Design review of the part built by this model. Coordinates are the model's own, in mm. Coordinates: 2 decimals unless noted, no trailing zeros. Write each loop counter-clockwise with the first axis right and the second up, starting at its lowest first coordinate (ties: lowest second). Pieces come first, ordered by that corner, then holes. Notation, with made-up numbers: (34.5, 3) - (70.5, 3) arc R28 ccw to (70.5, 21) - close; hole circle Ø8 at (10, -28.5). An arc over 180 degrees is marked (long way). Use a Markdown table: item, result.
from build123d import *

# Parameters (mm, degrees)
F1_DEPTH = 18
F3_D     = 8
F3_DEPTH = 11
F3_TIP   = 2.4034424761


# Not quite as in the source:
# - a feature names something its author has since deleted; it is built from what else it names


with BuildPart() as f1:
    # F0 (on Top) → F1 (new body)
    with BuildSketch(Plane.XY):
        with BuildLine():
            ThreePointArc((287.0371856283, 264.0258587081), (16.2714653094, 389.6604155116), (-264.0258587081, 287.0371856283))
            Line((-264.0258587081, 287.0371856283), (0, 0))
            Line((0, 0), (287.0371856283, 264.0258587081))
        make_face()
    extrude(amount=F1_DEPTH)

    # F3
    with Locations(Plane(origin=(0, 0, 0), x_dir=(1, 0, 0), z_dir=(0, 0, -1))):
        with Locations((-111.8492066751, -134.8916415726), (-52.612635811, -70.4922730022), (58.3064641387, -65.860505917), (122.7058327092, -125.097076781), (187.1052012796, -184.333647645), (-171.0857775391, -199.2910101431)):
            Hole(F3_D / 2, depth=F3_DEPTH)
            with Locations((0, 0, -(F3_DEPTH + F3_TIP / 2))):  # 118° drill point
                Cone(0, F3_D / 2, F3_TIP, mode=Mode.SUBTRACT)


solid = f1.part
(1) Take a section at B-B on y = 174. Write out the cut boundary in (x, z).
Determined:
| item | result |
|---|---|
| outline | (-160.05, 0) - (189.17, 0) - (189.17, 18) - (-160.05, 18) - close |
(2) Take a section at C-C on x = 44. Write out the cut boundary in (y, z), and give its area (3 significant figures).
Determined:
| item | result |
|---|---|
| outline | (40.47, 0) - (387.51, 0) - (387.51, 18) - (40.47, 18) - close |
| area | 6,250 mm2 |
(3) Take a section at A-A on z = 2.75. Write out the cut boundary in (x, y), and give its area (3 significant figures).
Determined:
| item | result |
|---|---|
| outline | (-264.03, 287.04) - (0, 0) - (287.04, 264.03) arc R390 ccw to start; hole circle Ø8 at (-171.09, 199.29); hole circle Ø8 at (-111.85, 134.89); hole circle Ø8 at (-52.61, 70.49); hole circle Ø8 at (58.31, 65.86); hole circle Ø8 at (122.71, 125.1); hole circle Ø8 at (187.11, 184.33) |
| area | 119,000 mm2 |
(4) For pin 1 (7 mm diameter, centred on x = -171.09, y = 199.29, fed in from -Z); pin 2 (1 mm diameter, centred on y = 301, z = 7, fed in from -X); pin 3 (5 mm diameter, centred on x = 187.11, y = 184.33, fed in from -Z), all flat-tipped, find the tip position at first contact; note any pin that passes through.
Determined:
| item | result |
|---|---|
| pin 1 | z = 11.3 |
| pin 2 | x = -248.6 |
| pin 3 | z = 11.9 |
(5) For L1, parallel to X at y = 123, z = 3.75; L2, parallel to X at y = 58.5, z = 6.75; L3, parallel to Y at x = 189.5, z = 8.5, list the stretches that pass through material, from the lowest coordinate up. Write a range as from..to.
Determined:
| item | result |
|---|---|
| L1 | -113.14..119.3, 126.11..133.72 |
| L2 | -53.81..63.6 |
| L3 | 174.31..181.13, 187.54..340.87 |
